Job drawing, mm, ordinate dimensions from the low corner. One solid piece. A direction names the side the tool comes from. Give positions to 0.01 mm unless a question says otherwise; leave off trailing zeros. Write each loop counter-clockwise with the first axis right and the second up, starting at its lowest first coordinate (ties: lowest second). Pieces come first, ordered by that corner, then holes. Notation, with made-up numbers: M 1,37.25 L 18,37.25 A32 ccw 18,70.25 Z; hole C 60,7.5 d9. An arc over 180 degrees is marked long. Answer as CSV lines item,"result". Start each with the question number.
1) Slice it at D-D, the plane y = 10.5. Give the cut face in (x, z).
2) Wall check: line 1 along X through (y, z) = (43.5, 104.5); line 2 along Z through (x, y) = (104, 50); line 3 along X through (y, z) = (57, 184). Give the ranges that are in metal, low to high. Write a range as from..to.
3) Slice it at B-B, the plane z = 126.5. Give the cut face in (x, y), plus the area to 3 significant figures.
4) Slice it at A-A, the plane x = 17.5. Give the cut face in (y, z), plus the area to 3 significant figures.
5) Pin check, flat tips, straight feed: pin 1 Ø2.5 at (x, z) = (2, 149) entering from +Y; pin 2 Ø3.5 at (x, z) = (15.5, 252) entering from -Y. Stop position of each tip, or through.
6) Slice it at C-C, the plane y = 45. Give the cut face in (x, z).
7) Tool access for the marked faces 1 and 2: list every direction of +Z, -Z, +X, -X, +Y, -Y with a clear straight run to the whole face (end or side of a thin tool).
8) Mould opens along X. For the marked faces 3, 4 and 5 say: pulls with the +X half, pulls with the -X half, needs draft (parallel to the pull), parting line crosses it, or undercut.
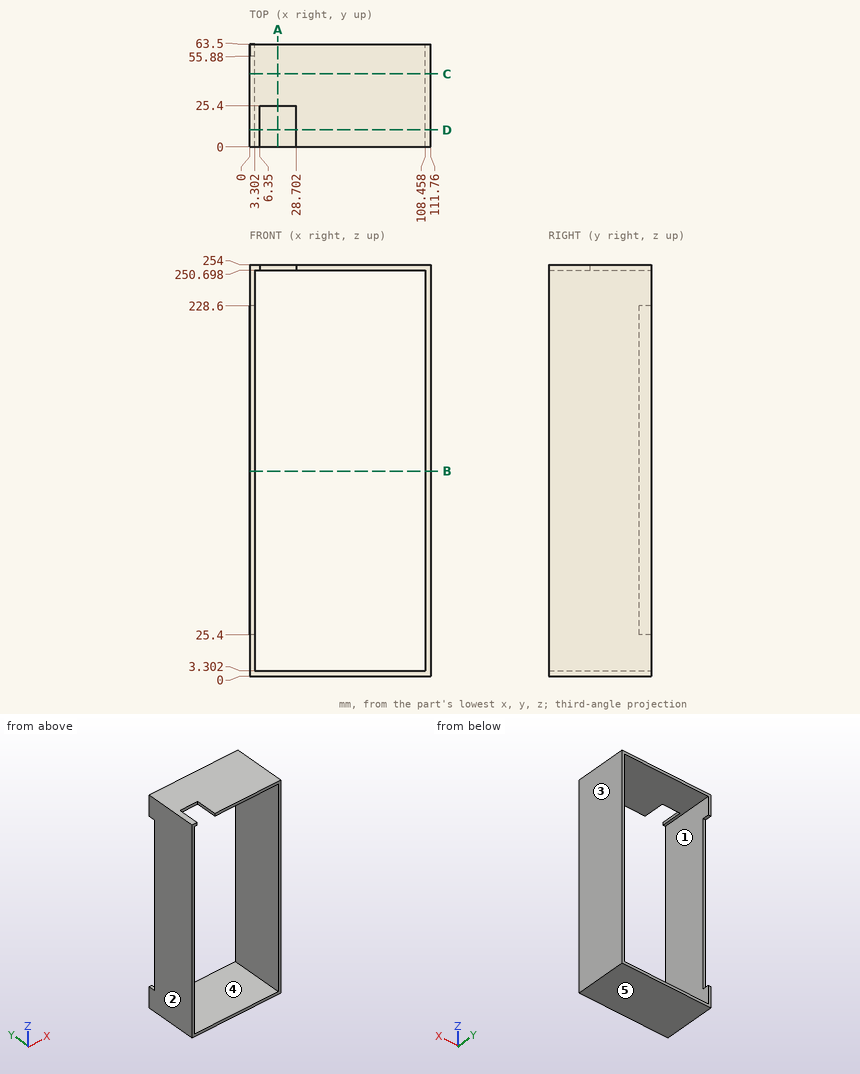
Found:
1,outline,"M 0,0 L 111.76,0 L 111.76,254 L 28.7,254 L 28.7,250.7 L 108.46,250.7 L 108.46,3.3 L 3.3,3.3 L 3.3,250.7 L 6.35,250.7 L 6.35,254 L 0,254 Z"
2,line 1,"0..3.3, 108.46..111.76"
2,line 2,"0..3.3, 250.7..254"
2,line 3,"108.46..111.76"
3,outline,"M 0,0 L 3.3,0 L 3.3,55.88 L 0,55.88 Z; M 108.46,0 L 111.76,0 L 111.76,63.5 L 108.46,63.5 Z"
3,area,"394 mm²"
4,outline,"M 0,0 L 63.5,0 L 63.5,3.3 L 0,3.3 Z; M 25.4,250.7 L 63.5,250.7 L 63.5,254 L 25.4,254 Z"
4,area,"335 mm²"
5,pin 1,"y = 55.88"
5,pin 2,"y = 25.4"
6,outline,"M 0,0 L 111.76,0 L 111.76,254 L 0,254 Z; hole M 3.3,3.3 L 108.46,3.3 L 108.46,250.7 L 3.3,250.7 Z"
7,face 1,"+Y, -Y"
7,face 2,"+Z, -Z, -X, +Y, -Y"
8,face 3,"pulls with the +X half"
8,face 4,"undercut"
8,face 5,"needs draft"
